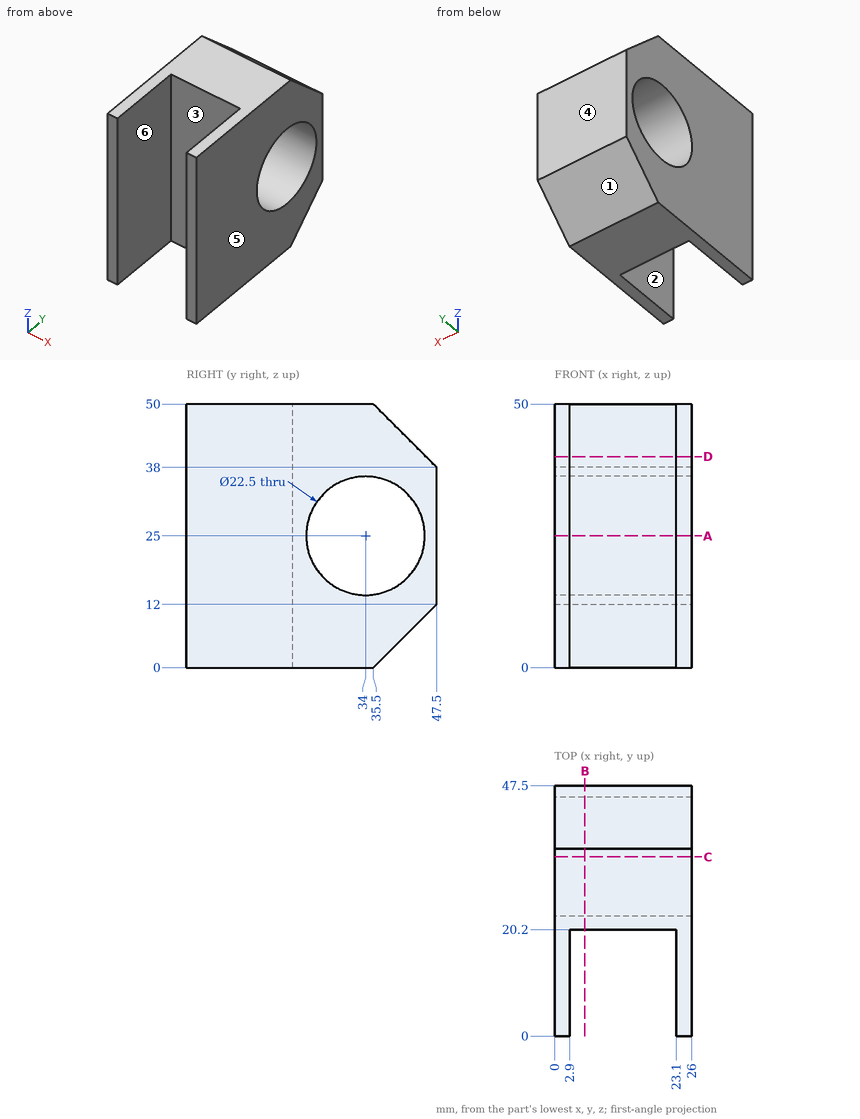
Geometry check sheet. Reference: drawing and pictorial views, mm from the part's lowest x, y, z. A direction names the side the tool comes from. Give positions to 0.01 mm unless a question says otherwise; leave off trailing zeros. Order: outer loops, then holes, each group sorted by start corner. A loop starts at its lowest first (then second) coordinate and runs counter-clockwise, first axis right, second up. Notation, with made-up numbers: M 75.5,-30 L 123.5,-30 A26 ccw 123.5,-8 Z; hole C 24.25,14.25 d10. An arc over 180 degrees is marked long. Use one line per item in the form item = value. Start each with the question number.
Q1. Mould release check, pull along X, two halves, no side actions. Record for the marked faces 3, 4, 5 and 6: +X half, -X half, draft (parallel to the pull), parting line (faces both ways), or undercut.
Q2. Section check B-B (x = 5.75). Enter the section's corners in (y, z), then the cut area to 3 significant figures.
Q3. Access from +Z, -Z, +X, -X, +Y, -Y to the whole of each face (thin tool, end or side, straight path). Record for the marked faces 1 and 2.
Q4. Go/stop test with flat-tipped pins: pin 1 Ø10 at (x, y) = (14.5, 42.5) entering from +Z; pin 2 Ø1.5 at (x, z) = (19, 42) entering from +Y. Record where each tip stops, or that it passes through.
Q5. Section check D-D (z = 40). Enter the section's corners in (x, y), then the cut area to 3 significant figures.
Q6. Scan lines: line 1 along X through (y, z) = (2.5, 47); line 2 along Z through (x, y) = (9, 34); line 3 along Y through (x, z) = (5.5, 25). Record each from-to range of solid material in increasing order. Write a range as [from, to].
Q7. Section check C-C (y = 34). Enter the section's corners in (x, z).
Q8. Section check A-A (z = 25). Enter the section's corners in (x, y), then the cut area to 3 significant figures.
Evaluation:
q1.face_3 = undercut
q1.face_4 = draft
q1.face_5 = +X half
q1.face_6 = undercut
q2.outline = M 20.2,0 L 35.5,0 L 47.5,12 L 47.5,38 L 35.5,50 L 20.2,50 Z; hole C 34,25 d22.5
q2.area = 823 mm2
q3.face_1 = -Z, +X, -X, +Y
q3.face_2 = +Z, -Z, -Y
q4.pin_1 = 48
q4.pin_2 = 44.25
q5.outline = M 0,0 L 2.9,0 L 2.9,20.2 L 23.1,20.2 L 23.1,0 L 26,0 L 26,45.5 L 0,45.5 Z
q5.area = 775 mm2
q6.line_1 = [0, 2.9], [23.1, 26]
q6.line_2 = [0, 13.75], [36.25, 50]
q6.line_3 = [20.2, 22.75], [45.25, 47.5]
q7.outline = M 0,0 L 26,0 L 26,13.75 L 0,13.75 Z; M 0,36.25 L 26,36.25 L 26,50 L 0,50 Z
q8.outline = M 0,0 L 2.9,0 L 2.9,20.2 L 23.1,20.2 L 23.1,0 L 26,0 L 26,22.75 L 0,22.75 Z; M 0,45.25 L 26,45.25 L 26,47.5 L 0,47.5 Z
q8.area = 242 mm2
